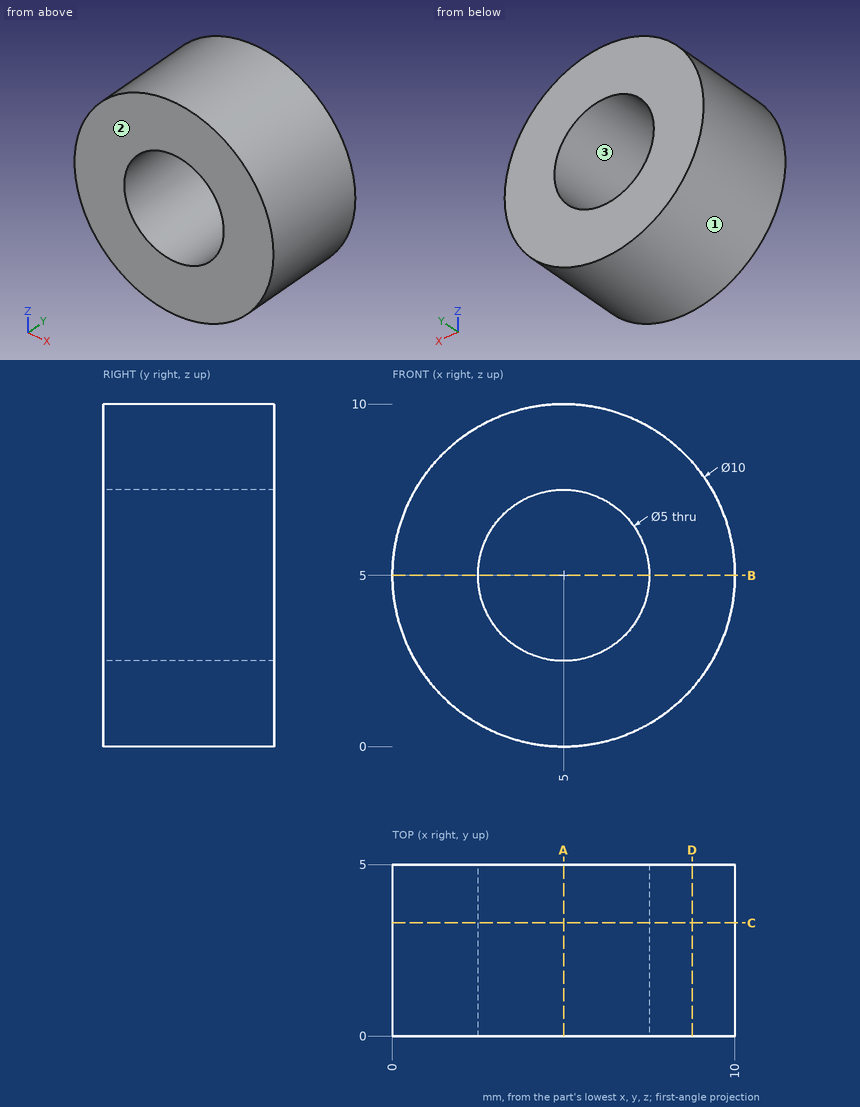
The drawing under review shows one solid part. Ordinate dimensions are in mm from its lowest x, y, z. Round coordinates to 2 decimals unless told otherwise and drop trailing zeros. Write each loop counter-clockwise with the first axis right and the second up, starting at its lowest first coordinate (ties: lowest second). Pieces come first, ordered by that corner, then holes. Notation, with made-up numbers: (10, -11) - (62, -11) arc R21 ccw to (62, 0) - close; hole circle Ø3 at (-2.5, -27). An arc over 180 degrees is marked (long way). Use one line per item in the form item = value.
Q1. Consider section D-D (x = 8.75). State the section outline as (y, z) points, and give its area (3 significant figures).
Answer key:
outline = (0, 1.69) - (5, 1.69) - (5, 8.31) - (0, 8.31) - close
area = 33.1 mm2
Q2. Consider section C-C (y = 3.3). State the section outline as (x, z) points, and give its area (3 significant figures).
Answer key:
outline = circle Ø10 at (5, 5); hole circle Ø5 at (5, 5)
area = 58.9 mm2
Q3. Consider section A-A (x = 5). State the section outline as (y, z) points, and give its area (3 significant figures).
Answer key:
outline = (0, 0) - (5, 0) - (5, 2.5) - (0, 2.5) - close; (0, 7.5) - (5, 7.5) - (5, 10) - (0, 10) - close
area = 25.0 mm2
Q4. Draft analysis for pull direction Z (two halves, no side actions). For the marked faces 1, 2 and 3, state which applies: +Z half, -Z half, draft (parallel to the pull), parting line (faces both ways), or undercut.
Answer key:
face_1 = parting line
face_2 = draft
face_3 = undercut
Q5. Insertion check: pin 1 Ø1.5 at (x, y) = (3.5, 1) entering from -Z. The pin has a flat end and moves straight along its axis. Give the tip position at first contact, or say it passes through.
Answer key:
pin_1 = 0.06
Q6. Consider section B-B (z = 5). State the section outline as (x, y) points.
Answer key:
outline = (0, 0) - (2.5, 0) - (2.5, 5) - (0, 5) - close; (7.5, 0) - (10, 0) - (10, 5) - (7.5, 5) - close
Q7. For line 1 (Z direction, x = 5, y = 1.55); line 2 (Z direction, x = 4.25, y = 2.8); line 3 (X direction, y = 0.2, z = 2.75), list the stretches that pass through material, from the lowest coordinate up. Write a range as [from, to].
Answer key:
line_1 = [0, 2.5], [7.5, 10]
line_2 = [0.06, 2.62], [7.38, 9.94]
line_3 = [0.53, 3.91], [6.09, 9.47]
